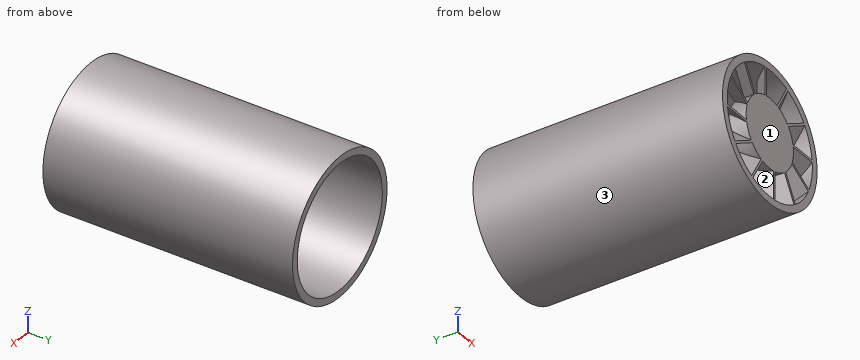
```python
from build123d import *

# Parameters (mm, degrees)
SKETCH1_R                            = 20
BOSS_EXTRUDE1_DEPTH                  = 10
SKETCH1_R_2                          = 40
SKETCH1_R_3                          = 36
BOSS_EXTRUDE1_2_DEPTH                = 10
BOSS_EXTRUDE2_REACH                  = 89.446
BOSS_EXTRUDE2_END_RADIUS             = 36
BOSS_EXTRUDE2_START                  = 30
BOSS_EXTRUDE2_DIRECTION_2_REACH      = 89.446
BOSS_EXTRUDE2_DIRECTION_2_END_RADIUS = 20
CIRPATTERN1_COUNT                    = 12
SKETCH5_R                            = 3.167731354
BOSS_EXTRUDE3_DEPTH                  = 10
SCALE1_SCALE                         = 0.75
SKETCH6_R                            = 30
SKETCH6_R_2                          = 27
BOSS_EXTRUDE4_DEPTH                  = 100


with BuildPart() as part:
    # Sketch1 → Boss-Extrude1 (new body)
    with BuildSketch(Plane(origin=(0, 0, 0), x_dir=(1, 0, 0), z_dir=(0, 1, 0))):
        with Locations(Location((0, 0, 0), (0, 0, 270))):
            Circle(SKETCH1_R)
    extrude(amount=BOSS_EXTRUDE1_DEPTH)


with BuildPart() as body_2:
    # Sketch1 → Boss-Extrude1 2 (new body)
    with BuildSketch(Plane(origin=(0, 0, 0), x_dir=(1, 0, 0), z_dir=(0, 1, 0))):
        with Locations(Location((0, 0, 0), (0, 0, 270))):
            Circle(SKETCH1_R_2)
        with Locations(Location((0, 0, 0), (0, 0, 270))):
            Circle(SKETCH1_R_3, mode=Mode.SUBTRACT)
    extrude(amount=BOSS_EXTRUDE1_2_DEPTH)


    add(part.part)  # Boss-Extrude2 merges part
    # Boss-Extrude2: up to this cylinder (the profile starts inside it)
    boss_extrude2_end = Plane(origin=(0, 5, 0), z_dir=(0, -1, 0)) * Cylinder(BOSS_EXTRUDE2_END_RADIUS, 251.892, mode=Mode.PRIVATE)
    # Sketch4 → Boss-Extrude2 (add, up to the surface)
    with BuildSketch(Plane(origin=(0, 0, 0), x_dir=(0, 0, -1), z_dir=(1, 0, 0)).offset(BOSS_EXTRUDE2_START), mode=Mode.PRIVATE) as boss_extrude2_sk1:
        Polygon((-4.262410526, 0), (4.031443844, 10), (5.315133993, 10), (-2.978720377, 0), align=None)
    boss_extrude2_tool1 = extrude(boss_extrude2_sk1.sketch, amount=BOSS_EXTRUDE2_REACH, mode=Mode.PRIVATE) & boss_extrude2_end
    boss_extrude2 = boss_extrude2_tool1.solids().sort_by_distance((30, 5, -0.526362))[0]
    add(boss_extrude2)

    # Boss-Extrude2 direction 2: up to this cylinder (the profile starts outside it)
    boss_extrude2_direction_2_end = Plane(origin=(0, 5, 0), z_dir=(0, -1, 0)) * Cylinder(BOSS_EXTRUDE2_DIRECTION_2_END_RADIUS, 219.892, mode=Mode.PRIVATE)
    # Sketch4 → Boss-Extrude2 direction 2 (add, up to the surface)
    with BuildSketch(Plane(origin=(0, 0, 0), x_dir=(0, 0, -1), z_dir=(1, 0, 0)).offset(BOSS_EXTRUDE2_START), mode=Mode.PRIVATE) as boss_extrude2_direction_2_sk1:
        Polygon((-4.262410526, 0), (4.031443844, 10), (5.315133993, 10), (-2.978720377, 0), align=None)
    boss_extrude2_direction_2_tool1 = extrude(boss_extrude2_direction_2_sk1.sketch, amount=-BOSS_EXTRUDE2_DIRECTION_2_REACH, mode=Mode.PRIVATE) - boss_extrude2_direction_2_end
    boss_extrude2_direction_2 = boss_extrude2_direction_2_tool1.solids().sort_by_distance((30, 5, -0.526362))[0]
    add(boss_extrude2_direction_2)
    boss_extrude2 = boss_extrude2 + boss_extrude2_direction_2  # both directions under the feature's name, for the pattern or mirror that repeats it

    # CirPattern1: Boss-Extrude2 ×12 about axis
    cirpattern1_axis = Axis((0, 0, 0), (0, 1, 0))
    for i in range(1, CIRPATTERN1_COUNT):
        add(boss_extrude2.rotate(cirpattern1_axis, i * 360 / CIRPATTERN1_COUNT))

    # Sketch5 → Boss-Extrude3 (add)
    with BuildSketch(Plane(origin=(0, 10, 0), x_dir=(1, 0, 0), z_dir=(0, 1, 0))):
        with Locations(Location((0, 0, 0), (0, 0, 270))):
            Circle(SKETCH5_R)
    extrude(amount=BOSS_EXTRUDE3_DEPTH)


with BuildPart() as body_2_1:
    # Scale1: scaled about (0, 0, 0)
    add(body_2.part.scale(SCALE1_SCALE))

    # Sketch6 → Boss-Extrude4 (add)
    with BuildSketch(Plane(origin=(0, 7.5, 0), x_dir=(1, 0, 0), z_dir=(0, 1, 0))):
        with Locations(Location((0, 0, 0), (0, 0, 270))):
            Circle(SKETCH6_R)
        with Locations(Location((0, 0, 0), (0, 0, 85.253793096))):
            Circle(SKETCH6_R_2, mode=Mode.SUBTRACT)
    extrude(amount=BOSS_EXTRUDE4_DEPTH)


solid = body_2_1.part
```
Check sheet for the modelled part. Datum: model origin and axes. Units: mm. Face numbers are marked on the shaded views. Give positions to 0.01 mm unless a question says otherwise; leave off trailing zeros. Write each loop counter-clockwise with the first axis right and the second up, starting at its lowest first coordinate (ties: lowest second). Pieces come first, ordered by that corner, then holes.
Item 1: Cross-section at A-A (z = 8). Enter the section's corners in (x, y).
Item 2: Cross-section at D-D (z = 1). Enter the section's corners in (x, y).
Item 3: Cross-section at B-B (x = -19.5). Enter the section's corners in (y, z).
Item 4: Cross-section at C-C (z = -19). Enter the section's corners in (x, y).
Item 5: Gauge pin test, flat ends, axial feed: pin 1 (3 mm diameter, centred on x = 10, y = 43.5, fed in from +Z); pin 2 (8 mm diameter, centred on x = 21, z = -0.5, fed in from -Y); pin 3 (8 mm diameter, centred on y = 86.5, z = -10, fed in from -X); pin 4 (10 mm diameter, centred on x = 6, z = 12, fed in from +Y). Record the tip position at first contact, or that the pin passes through.
Item 6: Draft check along X on the marked faces 1, 2 and 3. Enter one of: released by +X, released by -X, zero draft, split by the parting line, or undercut.
Item 7: Scan lines: L1, parallel to X at y = 38, z = 0; L2, parallel to Y at x = 4, z = -1; L3, parallel to X at y = 37, z = -23. Record each from-to range of solid material in increasing order.
Report:
1. outline: (-28.91, 0) - (-25.79, 0) - (-25.79, 107.5) - (-28.91, 107.5) - close; (-20.25, 0) - (-18.32, 0) - (-12.69, 3.4) - (-12.69, 0) - (12.69, 0) - (12.69, 1.99) - (21.83, 7.5) - (19.9, 7.5) - (12.69, 3.15) - (12.69, 7.5) - (-12.69, 7.5) - (-12.69, 4.56) - close; (25.79, 0) - (28.91, 0) - (28.91, 107.5) - (25.79, 107.5) - close
2. outline: (-29.98, 0) - (-26.98, 0) - (-26.98, 3.9) - (-14.97, 3.9) - (-14.97, 0) - (14.97, 0) - (14.97, 1.49) - (26.98, 1.49) - (26.98, 0) - (29.98, 0) - (29.98, 107.5) - (26.98, 107.5) - (26.98, 2.65) - (14.97, 2.65) - (14.97, 7.5) - (2.16, 7.5) - (2.16, 15) - (-2.16, 15) - (-2.16, 7.5) - (-14.97, 7.5) - (-14.97, 5.06) - (-26.98, 5.06) - (-26.98, 107.5) - (-29.98, 107.5) - close
3. outline: (0, -22.8) - (107.5, -22.8) - (107.5, -18.67) - (0, -18.67) - close; (0, -14.95) - (7.5, -7.77) - (7.5, -6.66) - (0, -13.84) - close; (0, -3.2) - (7.5, 3.02) - (7.5, 3.99) - (0, -2.23) - close; (0, 7.57) - (7.5, 14.75) - (7.5, 15.86) - (0, 8.68) - close; (0, 18.67) - (107.5, 18.67) - (107.5, 22.8) - (0, 22.8) - close
4. outline: (-23.22, 0) - (-19.18, 0) - (-19.18, 107.5) - (-23.22, 107.5) - close; (-15.57, 7.5) - (-8.39, 0) - (-7.28, 0) - (-14.46, 7.5) - close; (-3.99, 7.5) - (2.23, 0) - (3.2, 0) - (-3.02, 7.5) - close; (6.37, 7.5) - (13.55, 0) - (14.66, 0) - (7.48, 7.5) - close; (19.18, 0) - (23.22, 0) - (23.22, 107.5) - (19.18, 107.5) - close
5. pin 1: stops at z = 28.77
5. pin 2: stops at y = 0
5. pin 3: stops at x = -29.39
5. pin 4: stops at y = 7.5
6. face 1: zero draft
6. face 2: undercut
6. face 3: split by the parting line
7. L1: x = -30 to -27, 27 to 30
7. L2: y = 0 to 7.5
7. L3: x = -19.26 to -14.14, 14.14 to 19.26
